from build123d import *
from build123d import SkipClean  # not in build123d's __all__

# Parameters (mm, degrees)
F1_DEPTH = 2.8575


with BuildPart() as f1:
    # F0 (on Top) → F1 (new body, symmetric)
    with BuildSketch(Plane.XY):
        with BuildLine():
            ThreePointArc((0, -75.7864124179), (4, -79.7864124179), (0, -83.7864124179))
            Line((0, -83.7864124179), (0, -89.3016444676))
            ThreePointArc((0, -89.3016444676), (7.3191604153, -85.8666699597), (9.3539243357, -78.0417805136))
            Line((9.3539243357, -78.0417805136), (6.731, -63.9788508415))
            Line((6.731, -63.9788508415), (6.731, 0))
            Line((6.731, 0), (0, 0))
            Line((0, 0), (0, -75.7864124179))
        make_face()
    extrude(amount=F1_DEPTH, both=True)

    # F2: F1 across plane


with BuildPart() as f1_1:
    add(f1.part, clean=False)
    with SkipClean():  # cleaning this boolean's faces spoils the solid; the shape is the same uncleaned
        add(f1.part.mirror(Plane.YZ), clean=False)

    # F3: F1 across plane


with BuildPart() as f1_2:
    add(f1_1.part, clean=False)
    add(f1_1.part.mirror(Plane.XZ), clean=False)


solid = f1_2.part
Input: part model. Units: mm. Frame: model coordinates. A direction names the side the tool comes from. Round coordinates to 2 decimals unless told otherwise and drop trailing zeros. Order: outer loops, then holes, each group sorted by start corner. A loop starts at its lowest first (then second) coordinate and runs counter-clockwise, first axis right, second up. Notation, with made-up numbers: (37.5, 45.25) - (58.5, 45.25) arc R21 ccw to (58.5, 75.25) - close; hole circle Ø4 at (21, 33). An arc over 180 degrees is marked (long way). Answer as a JSON object with one key per item and string values. Group by question number.
(1) Cut plane A-A (z = 0). Return loops of the section in (x, y).
(2) Material intervals for probe 1 along X at (y, z) = (19, 1.7); probe 2 along Y at (x, z) = (-1.25, 0.2); probe 3 along X at (y, z) = (-75.5, -2.3), sorted ascending. Write a range as from..to.
(3) Cut plane B-B (y = -50). Return loops of the section in (x, z), then the cut area to 3 significant figures.
(4) Reachability of faces 1 (the face through (8.06, 71.11, 0.04)), 2 (the face through (-8.06, 71.11, 0.04)) from +Z, -Z, +X, -X, +Y, -Y: full face, straight path, thin tool, end or side. Return the list, or none.
(5) Pin query (flat end, axial travel): P1, Ø1.7, axis at y = 31, z = 0, coming from the +X side; P2, Ø1, axis at x = 1.5, z = 1.5, coming from the -Y side; P3, Ø3, axis at x = -5.5, z = 1, coming from the -Y side. Return the tip coordinate at first contact, or that it passes through.
Here are the results:
{
 "1": {"outline": "(-9.35, -78.04) arc R9.52 ccw (long way) to (9.35, -78.04) - (6.73, -63.98) - (6.73, 63.98) - (9.35, 78.04) arc R9.52 ccw (long way) to (-9.35, 78.04) - (-6.73, 63.98) - (-6.73, -63.98) - close; hole circle Ø8 at (0, -79.79); hole circle Ø8 at (0, 79.79)"},
 "2": {"probe 1": "x = -6.73..6.73", "probe 2": "y = -89.22..-83.59, -75.99..75.99, 83.59..89.22", "probe 3": "x = -8.88..8.88"},
 "3": {"outline": "(-6.73, -2.86) - (6.73, -2.86) - (6.73, 2.86) - (-6.73, 2.86) - close", "area": "76.9 mm^2"},
 "4": {"face 1": "+Z, -Z, +X", "face 2": "+Z, -Z, -X"},
 "5": {"P1": "stops at x = 6.73", "P2": "stops at y = -89.25", "P3": "stops at y = -88.42"}
}
